from build123d import *

# Parameters (mm, degrees)
CHAMFER1_SIZE      = 2.5
CUT_EXTRUDE1_START = -24
SKETCH3_R          = 11
SKETCH3_R_2        = 10.25
CUT_EXTRUDE1_DEPTH = 4
CHAMFER2_SIZE      = 1


with BuildPart() as part:
    # Sketch2 → Revolve1 (revolve)
    with BuildSketch(Plane(origin=(0, 0, 0), x_dir=(0, 0, -1), z_dir=(1, 0, 0)), mode=Mode.PRIVATE) as revolve1_sk:
        Polygon((0, 11), (24, 11), (29, 17.95), (53, 17.95), (53, 14.95), (30.537419245, 14.95), (25.537419245, 8), (0, 8), align=None)
    revolve(revolve1_sk.sketch.rotate(Axis((0, 0, 0), (0, 0, -1)), 90), axis=Axis((0, 0, 0), (0, 0, -1)))

    # Chamfer1
    chamfer1_edges = [part.edges().sort_by_distance(p)[0] for p in [
        (-17.95, 0, -53),
    ]]
    chamfer(chamfer1_edges, length=CHAMFER1_SIZE)

    # Sketch3 → Cut-Extrude1 (cut)
    with BuildSketch(Plane.XY.offset(CUT_EXTRUDE1_START)):
        Circle(SKETCH3_R)
        Circle(SKETCH3_R_2, mode=Mode.SUBTRACT)
    extrude(amount=CUT_EXTRUDE1_DEPTH, mode=Mode.SUBTRACT)

    # Chamfer2
    chamfer2_edges = [part.edges().sort_by_distance(p)[0] for p in [
        (-11, 0, 0),
    ]]
    chamfer(chamfer2_edges, length=CHAMFER2_SIZE)


solid = part.part
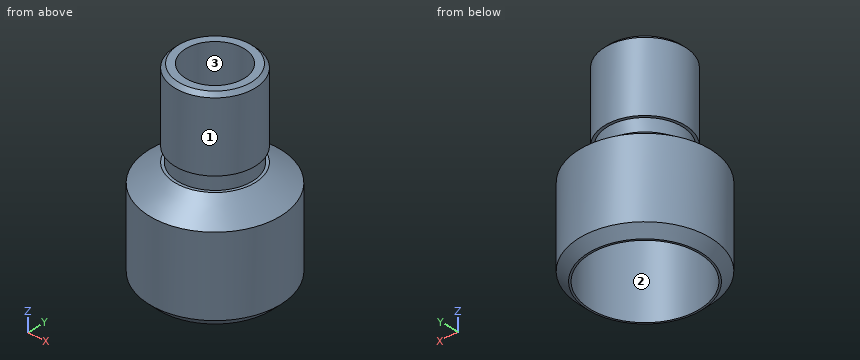
Build history of the part. All positions in model axes, mm. Face numbers are marked on the shaded views. Round coordinates to 2 decimals unless told otherwise and drop trailing zeros. Loops run counter-clockwise (first coordinate to the right, second up) from the corner with the lowest first, then second, coordinate; pieces in that order, holes last. Notation, with made-up numbers: (44, 25.5) -> (60, 25.5) arc R12 ccw to (60, 32.5) -> close; hole circle Ø10 at (19.5, -3.75). An arc over 180 degrees is marked (long way). Answer in a Markdown table with one row per item.
Item 1: Saw through at D-D (z = -41.5). Write the cut outline in (x, y).
Answers below:
| item | result |
|---|---|
| outline | circle Ø35.9 at (0, 0); hole circle Ø29.9 at (0, 0) |
Item 2: Saw through at C-C (z = -18). Write the cut outline in (x, y).
Answers below:
| item | result |
|---|---|
| outline | circle Ø22 at (0, 0); hole circle Ø16 at (0, 0) |
Item 3: Pin check, flat tips, straight feed: pin 1 (4 mm diameter, centred on x = -7.5, z = -34.5, fed in from -Y); pin 2 (6.5 mm diameter, centred on x = -2.5, y = 1, fed in from -Z); pin 3 (6 mm diameter, centred on y = 12.5, z = -12, fed in from +X); pin 4 (2 mm diameter, centred on x = 12, y = -7.5, fed in from +Z). Stop position of each tip, or through.
Answers below:
| item | result |
|---|---|
| pin 1 | stops at y = -17.09 |
| pin 2 | passes through |
| pin 3 | stops at x = 5.55 |
| pin 4 | stops at z = -25.55 |
Item 4: Saw through at A-A (x = 0). Write the cut outline in (y, z), and give its area (3 significant figures).
Answers below:
| item | result |
|---|---|
| outline | (-17.95, -50.5) -> (-15.45, -53) -> (-14.95, -53) -> (-14.95, -30.54) -> (-8, -25.54) -> (-8, 0) -> (-10, 0) -> (-11, -1) -> (-11, -20) -> (-10.25, -20) -> (-10.25, -24) -> (-11, -24) -> (-17.95, -29) -> close; (8, -25.54) -> (14.95, -30.54) -> (14.95, -53) -> (15.45, -53) -> (17.95, -50.5) -> (17.95, -29) -> (11, -24) -> (10.25, -24) -> (10.25, -20) -> (11, -20) -> (11, -1) -> (10, 0) -> (8, 0) -> close |
| area | 326 mm² |
Item 5: Drill centre lines: L1, parallel to Y at x = 0, z = -12.5; L2, parallel to Y at x = 0, z = -48; L3, parallel to Z at x = 10.5, y = -2. Where is each one in solid material? Low to high. Write a range as [from, to].
Answers below:
| item | result |
|---|---|
| L1 | y = [-11, -8], [8, 11] |
| L2 | y = [-17.95, -14.95], [14.95, 17.95] |
| L3 | z = [-27.47, -24], [-20, -0.69] |
Item 6: Mould opens along Y. For the marked faces 1, 2 and 3 say: +Y half, -Y half, draft (parallel to the pull), parting line (faces both ways), or undercut.
Answers below:
| item | result |
|---|---|
| face 1 | parting line |
| face 2 | undercut |
| face 3 | undercut |
